Source: CAD feature listing. Evaluate the final solid. Frame: model axes, mm. Give positions to 0.01 mm unless a question says otherwise; leave off trailing zeros. Order: outer loops, then holes, each group sorted by start corner. A loop starts at its lowest first (then second) coordinate and runs counter-clockwise, first axis right, second up. Notation, with made-up numbers: M 81,-30.75 L 120,-30.75 A16 ccw 120,-3.75 Z; hole C 54.25,60 d3. An arc over 180 degrees is marked long. Answer in a Markdown table with one row per item. Add a question column.
(1) Section query B-B, the plane x = -1. Return loops of the section in (y, z), plus the area to 3 significant figures.
(2) Material intervals for line 1 along Y through (x, z) = (-2, 62); line 2 along X through (y, z) = (5, 47), sorted ascending.
(3) Pin query (flat end, axial travel): P1, Ø1.7, axis at x = -1, z = 75.5, coming from the -Y side; P2, Ø1.9, axis at y = 84, z = 77, coming from the -X side. Return the tip coordinate at first contact, or that it passes through.
(4) Section query A-A, the plane z = 79.5. Return loops of the section in (x, y), plus the area to 3 significant figures.
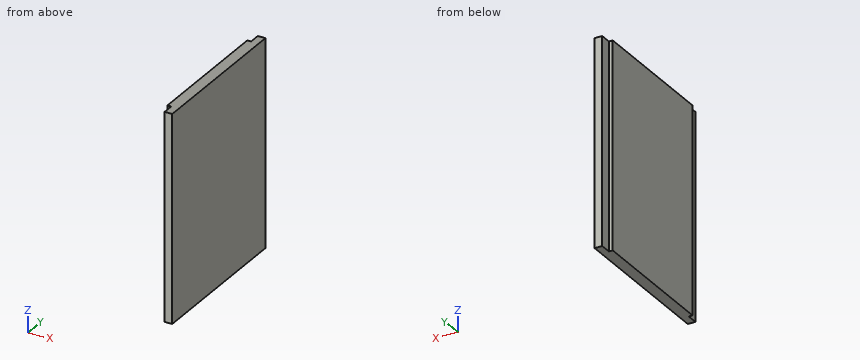
from build123d import *

# Parameters (mm, degrees)
F0_W     = 88.9
F0_H     = 114.3
F1_DEPTH = 4.2418
F2_W     = 76.2
F2_H     = 114.3
F3_DEPTH = 2.11582


# Not quite as in the source:
# - a feature names something its author has since deleted; it is built from what else it names


with BuildPart() as f1:
    # F0 (on Right) → F1 (new body)
    with BuildSketch(Plane.YZ):
        with Locations((44.45, 57.15)):
            Rectangle(F0_W, F0_H)
    extrude(amount=F1_DEPTH)

    # F2 (on Right) → F3 (join)
    with BuildSketch(Plane.YZ):
        with Locations((44.45, 57.15)):
            Rectangle(F2_W, F2_H)
    extrude(amount=-F3_DEPTH)


solid = f1.part
Values follow:
| question | item | result |
|---|---|---|
| 1 | outline | M 6.35,0 L 82.55,0 L 82.55,114.3 L 6.35,114.3 Z |
| 1 | area | 8,710 mm² |
| 2 | line 1 | y = 6.35 to 82.55 |
| 2 | line 2 | x = 0 to 4.24 |
| 3 | P1 | stops at y = 6.35 |
| 3 | P2 | stops at x = 0 |
| 4 | outline | M -2.12,6.35 L 0,6.35 L 0,0 L 4.24,0 L 4.24,88.9 L 0,88.9 L 0,82.55 L -2.12,82.55 Z |
| 4 | area | 538 mm² |
